Verification items for the finished model (mm, model axes). A direction names the side the tool comes from. Round coordinates to 2 decimals unless told otherwise and drop trailing zeros. Order: outer loops, then holes, each group sorted by start corner. A loop starts at its lowest first (then second) coordinate and runs counter-clockwise, first axis right, second up. Notation, with made-up numbers: M 35.25,20.5 L 43.25,20.5 A22 cw 43.25,58.5 Z; hole C 67,8 d2. An arc over 180 degrees is marked long. Write item = value, one per line. Start each with the question number.
from build123d import *

# Parameters (mm, degrees)
F1_DEPTH = 10
F3_DEPTH = 10
F4_COUNT = 18


with BuildPart() as f1:
    # F0 (on Front) → F1 (new body)
    with BuildSketch(Plane.XZ):
        with BuildLine():
            ThreePointArc((-1.1334270023, 9.9355595328), (-6.6582929485, -7.461041148), (10, 0))
            ThreePointArc((10, 0), (7.461041148, 6.6582929485), (1.1334270023, 9.9355595328))
            ThreePointArc((1.1334270023, 9.9355595328), (0, 10), (-1.1334270023, 9.9355595328))
        make_face()
    extrude(amount=-F1_DEPTH)

    # F2 (on face) → F3 (join)
    with BuildSketch(Plane.XZ):
        with BuildLine():
            Line((-0.906307787, 10.4226182617), (-1.1334270023, 9.9355595328))
            ThreePointArc((-1.1334270023, 9.9355595328), (0, 9.5833893877), (1.1334270023, 9.9355595328))
            Line((1.1334270023, 9.9355595328), (0.906307787, 10.4226182617))
            ThreePointArc((0.906307787, 10.4226182617), (0.5372996083, 10.8433914458), (0, 11))
            ThreePointArc((0, 11), (-0.5372996083, 10.8433914458), (-0.906307787, 10.4226182617))
        make_face()
    extrude(amount=-F3_DEPTH)

    # F4: F1 ×18 about axis
    f4_axis = Axis((0, 0, 0), (0, -1, 0))


with BuildPart() as f1_1:
    add(f1.part)
    for i in range(1, F4_COUNT):
        add(f1.part.rotate(f4_axis, i * 360 / F4_COUNT))


solid = f1_1.part
1) Cross-section at B-B, the plane z = 3.25. Enter the section's corners in (x, y).
2) Scan lines: probe 1 along X at (y, z) = (5.5, -7.75); probe 2 along Z at (x, y) = (6.5, 9.25); probe 3 along X at (y, z) = (8.5, -0.5). Record each from-to range of solid material in increasing order.
3) Release check for a two-part mould opening along Z. For faces 4 (the cylindrical face through (-9.4, 4.93, -3.41)), 5 (the cylindrical face through (-4.993, 4.93, 8.665)), 6 (the cylindrical face through (-1.745, 4.93, -9.847)) record: pulls with the +Z half, pulls with the -Z half, needs draft (parallel to the pull), parting line crosses it, or undercut.
4) Access from +Z, -Z, +X, -X, +Y, -Y to the whole of each face (thin tool, end or side, straight path). Record for faces 1 (the cylindrical face through (1.745, 4.93, 9.847)), 2 (the cylindrical face through (-5.007, 4.93, -8.656)), 3 (the cylindrical face through (9.394, 4.93, -3.428)).
5) Gauge pin test, flat ends, axial feed: P1, Ø1, axis at x = 6.5, y = 8.5, coming from the +Z side; P2, Ø4, axis at x = -4, y = 5.5, coming from the -Z side; P3, Ø1, axis at x = -4.5, y = 6, coming from the -Z side. Record the tip position at first contact, or that the pin passes through.
6) Cross-section at A-A, the plane x = -5. Enter the section's corners in (y, z).
Geometry results:
q1.outline = M -9.46,0 L 9.46,0 L 9.46,10 L -9.46,10 Z
q2.probe_1 = -7.42 to 7.42
q2.probe_2 = -8.66 to 8.66
q2.probe_3 = -9.99 to 9.99
q3.face_4 = undercut
q3.face_5 = pulls with the +Z half
q3.face_6 = pulls with the -Z half
q4.face_1 = +Z, +Y, -Y
q4.face_2 = -Z, +Y, -Y
q4.face_3 = +X, +Y, -Y
q5.P1 = 8.66
q5.P2 = -10.4
q5.P3 = -10.21
q6.outline = M 0,-8.66 L 10,-8.66 L 10,8.66 L 0,8.66 Z
